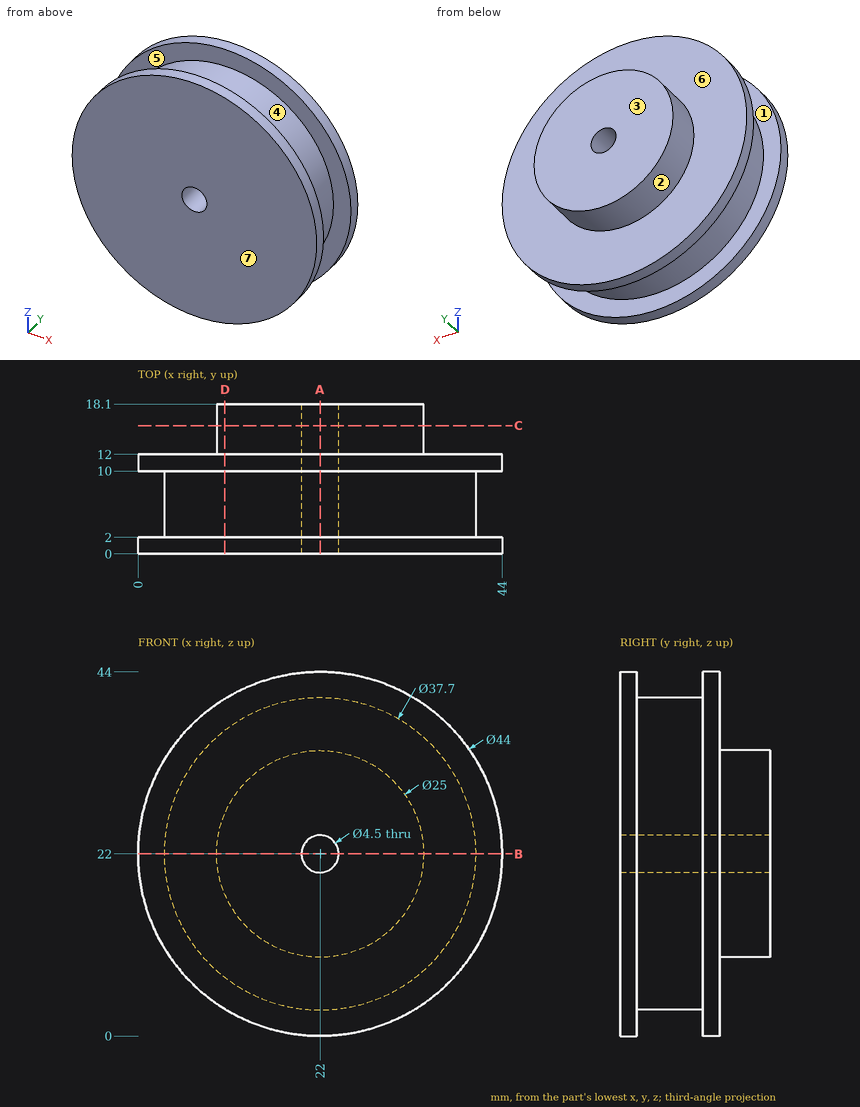
Input: dimensioned drawing with shaded views. Units: mm. Origin: part minimum x, y, z. A direction names the side the tool comes from. Coordinates: 2 decimals unless noted, no trailing zeros. Order: outer loops, then holes, each group sorted by start corner. A loop starts at its lowest first (then second) coordinate and runs counter-clockwise, first axis right, second up. Notation, with made-up numbers: (72.25, 30.5) - (108.25, 30.5) arc R34 ccw to (108.25, 62.5) - close; hole circle Ø6 at (10, 21.25). An arc over 180 degrees is marked (long way). Put each result on its own line as item: value.
1. Contact query for flat-ended pins moving along their axis: pin 1 Ø5 at (y, z) = (6, 36) entering from +X; pin 2 Ø1.5 at (y, z) = (3.5, 14) entering from +X; pin 3 Ø2 at (y, z) = (14, 14) entering from -X. Output: stop coordinate, or through.
Report:
pin 1: stops at x = 36.94
pin 2: stops at x = 39.4
pin 3: stops at x = 11.64
2. Cut plane D-D on x = 10.5. Return the cut outline in (y, z) (3 decimals), then the cut area to 3 significant figures.
Report:
outline: (0, 3.245) - (2, 3.245) - (2, 7.064) - (10, 7.064) - (10, 3.245) - (12, 3.245) - (12, 17.101) - (18.1, 17.101) - (18.1, 26.899) - (12, 26.899) - (12, 40.755) - (10, 40.755) - (10, 36.936) - (2, 36.936) - (2, 40.755) - (0, 40.755) - close
area: 449 mm2
3. Cut plane B-B on z = 22. Return the cut outline in (x, y), then the cut area to 3 significant figures.
Report:
outline: (0, 0) - (19.75, 0) - (19.75, 18.1) - (9.5, 18.1) - (9.5, 12) - (0, 12) - (0, 10) - (3.15, 10) - (3.15, 2) - (0, 2) - close; (24.25, 0) - (44, 0) - (44, 2) - (40.85, 2) - (40.85, 10) - (44, 10) - (44, 12) - (34.5, 12) - (34.5, 18.1) - (24.25, 18.1) - close
area: 549 mm2
4. Reachability of the marked faces 5, 6 and 7 from +Z, -Z, +X, -X, +Y, -Y: full face, straight path, thin tool, end or side. Return the list, or none.
Report:
face 5: none
face 6: +Y
face 7: +Z, -Z, +X, -X, -Y
5. Line query: line 1 along Y through (x, z) = (36.5, 6); line 2 along Z through (x, y) = (22, 12.5); line 3 along Y through (x, z) = (36.5, 33). Output: solid intervals per line, ascending.
Report:
line 1: y = 0 to 2, 10 to 12
line 2: z = 9.5 to 19.75, 24.25 to 34.5
line 3: y = 0 to 12
6. Cut plane A-A on x = 22. Return the cut outline in (y, z).
Report:
outline: (0, 0) - (2, 0) - (2, 3.15) - (10, 3.15) - (10, 0) - (12, 0) - (12, 9.5) - (18.1, 9.5) - (18.1, 19.75) - (0, 19.75) - close; (0, 24.25) - (18.1, 24.25) - (18.1, 34.5) - (12, 34.5) - (12, 44) - (10, 44) - (10, 40.85) - (2, 40.85) - (2, 44) - (0, 44) - close
7. Draft query along Y for the marked faces 1, 2, 3 and 4. Return one class per face: pulls with the +Y half, pulls with the -Y half, needs draft (parallel to the pull), parting line crosses it, or undercut.
Report:
face 1: undercut
face 2: needs draft
face 3: pulls with the +Y half
face 4: undercut
8. Cut plane C-C on y = 15.5. Return the cut outline in (x, z), then the cut area to 3 significant figures.
Report:
outline: circle Ø25 at (22, 22); hole circle Ø4.5 at (22, 22)
area: 475 mm2
